```python
from build123d import *

# Parameters (mm, degrees)
SKETCH1_W           = 57.15
SKETCH1_H           = 95.25
SKETCH1_R           = 1.375
BOSS_EXTRUDE1_DEPTH = 1.5875
SKETCH1_3_W         = 57.15
SKETCH1_3_H         = 95.25
SKETCH1_3_W_2       = 53.975
SKETCH1_3_H_2       = 92.075
BOSS_EXTRUDE2_DEPTH = 19.05
SKETCH3_R           = 2.05
BOSS_EXTRUDE5_DEPTH = 6.35
FILLET1_R           = 2.54


with BuildPart() as part:
    # Sketch1 → Boss-Extrude1 (new body)
    with BuildSketch(Plane(origin=(0, 0, 0), x_dir=(1, 0, 0), z_dir=(0, 1, 0))):
        Rectangle(SKETCH1_W, SKETCH1_H)
        with Locations((-17.4625, 39.6875)):
            Circle(SKETCH1_R, mode=Mode.SUBTRACT)
        with Locations((17.4625, 39.6875)):
            Circle(SKETCH1_R, mode=Mode.SUBTRACT)
        with Locations((-17.4625, -39.6875)):
            Circle(SKETCH1_R, mode=Mode.SUBTRACT)
        with Locations((17.4625, -39.6875)):
            Circle(SKETCH1_R, mode=Mode.SUBTRACT)
    extrude(amount=-BOSS_EXTRUDE1_DEPTH)

    # Sketch1_3 → Boss-Extrude2 (add)
    with BuildSketch(Plane(origin=(0, 0, 0), x_dir=(1, 0, 0), z_dir=(0, 1, 0))):
        Rectangle(SKETCH1_3_W, SKETCH1_3_H)
        Rectangle(SKETCH1_3_W_2, SKETCH1_3_H_2, mode=Mode.SUBTRACT)
    extrude(amount=BOSS_EXTRUDE2_DEPTH)

    # Sketch3 → Boss-Extrude5 (add)
    with BuildSketch(Plane.XZ.offset(1.5875)):
        with BuildLine():
            Line((28.575, 15.875), (34.925, 15.875))
            ThreePointArc((34.925, 15.875), (38.1, 19.05), (34.925, 22.225))
            Line((34.925, 22.225), (28.575, 22.225))
            Line((28.575, 22.225), (28.575, 15.875))
        make_face()
        with Locations((34.925, 19.05)):
            Circle(SKETCH3_R, mode=Mode.SUBTRACT)
        with BuildLine():
            Line((34.925, -15.875), (28.575, -15.875))
            Line((28.575, -15.875), (28.575, -22.225))
            Line((28.575, -22.225), (34.925, -22.225))
            ThreePointArc((34.925, -22.225), (38.1, -19.05), (34.925, -15.875))
        make_face()
        with Locations((34.925, -19.05)):
            Circle(SKETCH3_R, mode=Mode.SUBTRACT)
    extrude(amount=-BOSS_EXTRUDE5_DEPTH)

    # Fillet1
    fillet1_edges = [part.edges().sort_by_distance(p)[0] for p in [
        (28.575, 1.5875, -22.225),
        (28.575, 1.5875, -15.875),
        (28.575, 1.5875, 15.875),
        (28.575, 1.5875, 22.225),
    ]]
    fillet(fillet1_edges, radius=FILLET1_R)


solid = part.part
```
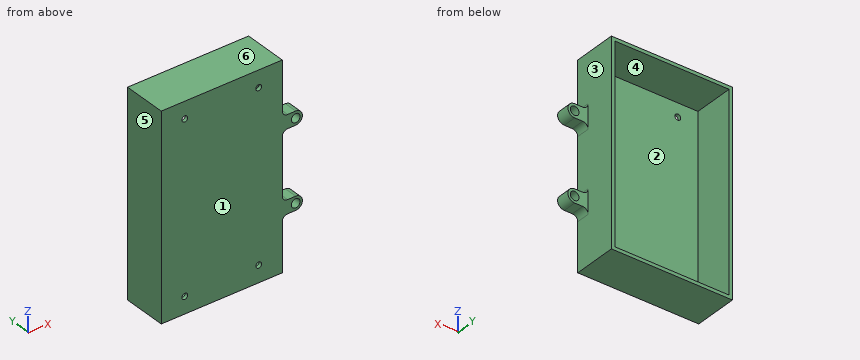
Here's how the part is built. I have some questions about the finished solid (model axes, mm). Face numbers are marked on the shaded views. A direction names the side the tool comes from. Round coordinates to 2 decimals unless told otherwise and drop trailing zeros. Order: outer loops, then holes, each group sorted by start corner. A loop starts at its lowest first (then second) coordinate and runs counter-clockwise, first axis right, second up. Notation, with made-up numbers: M 64,-25.75 L 83,-25.75 A25 ccw 83,-6.75 Z; hole C 19.5,-35 d11. An arc over 180 degrees is marked long. Answer as CSV lines item,"result".
Item 1: For pin 1 (10 mm diameter, centred on y = 2, z = -5.5, fed in from +X) (3 decimals); pin 2 (3 mm diameter, centred on x = 33.5, y = 2, fed in from -Z) (3 decimals); pin 3 (4 mm diameter, centred on x = 32.5, y = 1.5, fed in from -Z), each with a flat end and sliding along its axis, tell me the tip position at first contact or that it passes through.
From the geometry:
pin 1,"x = 28.575"
pin 2,"z = -22.225"
pin 3,"z = -22.3"
Item 2: Please list where these lines run through material, in increasing order: L1, parallel to Z at x = -12, y = 15 (1 decimal); L2, parallel to X at y = 5, z = 0 (1 decimal); L3, parallel to Y at x = -23.5, z = 39.5. Write a range as [from, to].
From the geometry:
L1,"[-47.6, -46], [46, 47.6]"
L2,"[-28.6, -27], [27, 28.6]"
L3,"[-1.59, 0]"
Item 3: Which directions (+Z, -Z, +X, -X, +Y, -Y) give clear straight access to the entire face, cutting with the end or side of a thin tool? Please do the marked faces 1, 2 and 3.
From the geometry:
face 1,"+Z, -Z, +X, -X, -Y"
face 2,"+Y"
face 3,"+X, +Y"
Item 4: Imagine slicing it at A-A on y = 7.75. List the corners of the cut face in (x, z) for me (1 decimal), and give its area (3 significant figures).
From the geometry:
outline,"M -28.6,-47.6 L 28.6,-47.6 L 28.6,47.6 L -28.6,47.6 Z; hole M -27,-46 L 27,-46 L 27,46 L -27,46 Z"
area,"474 mm2"
Item 5: We'd pull the mould along Z, two halves only. Please class the marked faces 4, 5 and 6: +Z half, -Z half, draft (parallel to the pull), parting line (faces both ways), or undercut.
From the geometry:
face 4,"undercut"
face 5,"draft"
face 6,"+Z half"
